from build123d import *

# Parameters (mm, degrees)
EXTRUDE1_DEPTH               = 30
SKETCH2_W                    = 4.1
SKETCH2_H                    = 60
CUT_FOR_WALKER_CHASSIS_DEPTH = 41.368552117
F_4_2_4_2_DIAMETER_HOLE1_D   = 4.2
M4X0_7_TAPPED_HOLE1_D        = 4
SKETCH7_R                    = 1.6
CUT_EXTRUDE1_DEPTH           = 39.598056946
CUT_EXTRUDE_2_DEPTH          = 10


with BuildPart() as part:
    # Sketch1 → Extrude1 (new, symmetric)
    with BuildSketch(Plane.XY):
        Polygon((0, 0), (0, 19.1), (3.3, 19.1), (3.3, 3.3), (19.1, 3.3), (19.1, 0), align=None)
    extrude(amount=EXTRUDE1_DEPTH, both=True)

    # Sketch2 → Cut for walker chassis (cut, through all)
    with BuildSketch(Plane.XZ):
        with Locations((17.05, 0)):
            Rectangle(SKETCH2_W, SKETCH2_H)
    extrude(amount=-CUT_FOR_WALKER_CHASSIS_DEPTH, mode=Mode.SUBTRACT)

    # Ø4.2 (4.2) Diameter Hole1 (through all)
    with Locations(Plane.ZY):
        with Locations((-19.5, 7.18), (19.5, 7.18)):
            Hole(F_4_2_4_2_DIAMETER_HOLE1_D / 2)

    # M4x0.7 Tapped Hole1 (through all)
    with Locations(Plane.XZ):
        with Locations((10, 25), (10, -25)):
            Hole(M4X0_7_TAPPED_HOLE1_D / 2)

    # Sketch7 → Cut-Extrude1 (cut, through all)
    with BuildSketch(Plane.XZ):
        with Locations((7.25, -12)):
            Circle(SKETCH7_R)
        with Locations((7.25, 12)):
            Circle(SKETCH7_R)
    extrude(amount=-CUT_EXTRUDE1_DEPTH, mode=Mode.SUBTRACT)

    # Эскиз3 → Вырез-Вытянуть2 (cut)
    with BuildSketch(Plane(origin=(0, 0, 0), x_dir=(0, 0, -1), z_dir=(1, 0, 0))):
        with BuildLine():
            Line((-30, 19.1), (-30, 4.1))
            ThreePointArc((-30, 4.1), (-25.606601718, 14.706601718), (-15, 19.1))
            Line((-15, 19.1), (-30, 19.1))
        make_face()
    cut_extrude_2 = extrude(amount=CUT_EXTRUDE_2_DEPTH, mode=Mode.SUBTRACT)

    # Зеркальное отражение1: Вырез-Вытянуть2 across plane
    add(cut_extrude_2.mirror(Plane.XY), mode=Mode.SUBTRACT)


solid = part.part
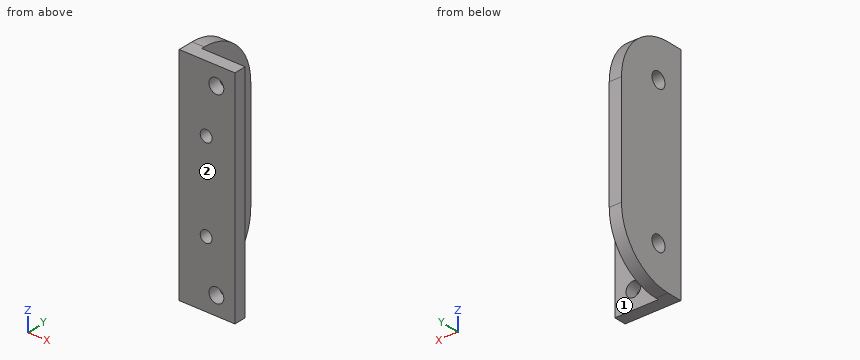
Input: part model. Units: mm. Frame: model coordinates. Face numbers are marked on the shaded views. A direction names the side the tool comes from. Give positions to 0.01 mm unless a question says otherwise; leave off trailing zeros. Loops run counter-clockwise (first coordinate to the right, second up) from the corner with the lowest first, then second, coordinate; pieces in that order, holes last. Notation, with made-up numbers: (39, -9) -> (90, -9) arc R16 ccw to (90, 14) -> close; hole circle Ø6 at (54.5, -27.75). An arc over 180 degrees is marked (long way). Answer as a JSON object with one key per item and string values. Group by question number.
Item 1: Line query: probe 1 along Z at (x, y) = (10, 0.9); probe 2 along Z at (x, y) = (7.25, 2.45); probe 3 along Y at (x, z) = (1, -15.5). Output: solid intervals per line, ascending.
Item 2: Pin query (flat end, axial travel): P1, Ø1, axis at x = 2.5, z = 0.5, coming from the -Y side; P2, Ø6.5, axis at x = 10, z = -25, coming from the +Y side; P3, Ø3, axis at x = 7.25, z = -12, coming from the +Y side; P4, Ø2, axis at y = 14.5, z = -9, coming from the +X side. Return the tip coordinate at first contact, or that it passes through.
Item 3: Cut plane D-D, the plane z = -20. Return the cut outline in (x, y).
Item 4: Cut plane B-B, the plane x = 7.25. Return the cut outline in (y, z), and give its area (3 significant figures).
Item 5: Cut plane C-C, the plane x = 2.25. Return the cut outline in (y, z), and give its area (3 significant figures).
Item 6: Reachability of the marked faces 1 and 2 from +Z, -Z, +X, -X, +Y, -Y: full face, straight path, thin tool, end or side. Return the list, or none.
Item 7: Cut plane A-A, the plane z = -12. Return the cut outline in (x, y), and give its area (3 significant figures).
Checks:
{
 "1": {"probe 1": "z = -30 to -27, -23 to 23, 27 to 30", "probe 2": "z = -30 to -13.6, -10.4 to 10.4, 13.6 to 30", "probe 3": "y = 0 to 19.09"},
 "2": {"P1": "stops at y = 0", "P2": "stops at y = 3.3", "P3": "passes through", "P4": "stops at x = 3.3"},
 "3": {"outline": "(0, 0) -> (15, 0) -> (15, 3.3) -> (3.3, 3.3) -> (3.3, 5.14) -> (0, 5.14) -> close; (0, 9.22) -> (3.3, 9.22) -> (3.3, 18.24) -> (0, 18.24) -> close"},
 "4": {"outline": "(0, -30) -> (3.3, -30) -> (3.3, -13.6) -> (0, -13.6) -> close; (0, -10.4) -> (3.3, -10.4) -> (3.3, 10.4) -> (0, 10.4) -> close; (0, 13.6) -> (3.3, 13.6) -> (3.3, 30) -> (0, 30) -> close", "area": "177 mm²"},
 "5": {"outline": "(0, -30) -> (4.1, -30) arc R15 ccw to (19.1, -15) -> (19.1, 15) arc R15 ccw to (4.1, 30) -> (0, 30) -> close; hole circle Ø4.2 at (7.18, -19.5); hole circle Ø4.2 at (7.18, 19.5)", "area": "1,020 mm²"},
 "6": {"face 1": "+Z, -Z, +X, +Y", "face 2": "+Z, -Z, +X, -X, -Y"},
 "7": {"outline": "(0, 0) -> (5.65, 0) -> (5.65, 3.3) -> (3.3, 3.3) -> (3.3, 19.1) -> (0, 19.1) -> close; (8.85, 0) -> (15, 0) -> (15, 3.3) -> (8.85, 3.3) -> close", "area": "91.1 mm²"}
}
